from build123d import *
from build123d.topology import SkipClean

# Parameters (mm, degrees)
SKETCH_1_R          = 1
EXTRUDE_1_DEPTH     = 3
SKETCH_2_R          = 1
EXTRUDE_2_DEPTH     = 3
EXTRUDE_START       = -3
SKETCH_2_5_R        = 1
EXTRUDE_4_DEPTH     = 3.5
SKETCH_1_6_R        = 1.75
CUT_EXTRUDE_2_DEPTH = 4.5


with BuildPart() as part:
    # 草图1 → 凸台-拉伸1 (new body)
    with BuildSketch(Plane.XY):
        with BuildLine():
            Line((-16.25, -32.145825623), (16.25, -32.145825623))
            ThreePointArc((16.25, -32.145825623), (20.25, -28.145825623), (16.25, -24.145825623))
            Line((16.25, -24.145825623), (0, -24.145825623))
            Line((0, -24.145825623), (-16.25, -24.145825623))
            ThreePointArc((-16.25, -24.145825623), (-20.25, -28.145825623), (-16.25, -32.145825623))
        make_face()
        with Locations((-16.25, -28.145825623)):
            Circle(SKETCH_1_R, mode=Mode.SUBTRACT)
        with Locations((16.25, -28.145825623)):
            Circle(SKETCH_1_R, mode=Mode.SUBTRACT)
    extrude(amount=EXTRUDE_1_DEPTH)

    # 草图2 → 凸台-拉伸2 (add)
    with BuildSketch(Plane(origin=(0, 0, 0), x_dir=(-1, 0, 0), z_dir=(0, 0, -1))):
        with BuildLine():
            ThreePointArc((-16.356032043, -101.464832065), (-12.998767478, -105.201322829), (-8.636789042, -102.71019202))
            Line((-8.636789042, -102.71019202), (19.97488875, -29.603633498))
            ThreePointArc((19.97488875, -29.603633498), (14.792192125, -31.870714373), (12.52511125, -26.688017748))
            Line((12.52511125, -26.688017748), (-8.745712257, -81.037738685))
            Line((-8.745712257, -81.037738685), (-9.274078909, -83.991512561))
            Line((-9.274078909, -83.991512561), (-12.255645749, -27.933377702))
            ThreePointArc((-12.255645749, -27.933377702), (-16.037552079, -32.140179874), (-20.244354251, -28.358273544))
            Line((-20.244354251, -28.358273544), (-16.356032043, -101.464832065))
        make_face()
        with Locations((-12.361677792, -101.252384145)):
            Circle(SKETCH_2_R, mode=Mode.SUBTRACT)
    extrude(amount=-EXTRUDE_2_DEPTH)

    # 草图2<5> → 凸台-拉伸4 (add)
    # profile 1 of 2: a face of its own
    with SkipClean():  # the faces are left unmerged after this step: merging them gives an invalid solid
        with BuildSketch(Plane(origin=(0, 0, 0), x_dir=(-1, 0, 0), z_dir=(0, 0, -1)).offset(EXTRUDE_START)):
            with BuildLine():
                ThreePointArc((-16.25, -24.145825623), (-19.152567112, -25.393534912), (-20.244354251, -28.358273544))
                ThreePointArc((-20.244354251, -28.358273544), (-19.002290711, -31.048392735), (-16.25, -32.145825623))
                ThreePointArc((-16.25, -32.145825623), (-13.421572875, -30.974252748), (-12.25, -28.145825623))
                ThreePointArc((-12.25, -28.145825623), (-12.251411686, -28.039564161), (-12.255645749, -27.933377702))
                ThreePointArc((-12.255645749, -27.933377702), (-13.497709289, -25.243258511), (-16.25, -24.145825623))
            make_face()
            with Locations(Location((-16.25, -28.145825623, 0), (0, 0, 180))):
                Circle(SKETCH_2_5_R, mode=Mode.SUBTRACT)
        # profile 2 of 2: a face of its own
        with BuildSketch(Plane(origin=(0, 0, 0), x_dir=(-1, 0, 0), z_dir=(0, 0, -1)).offset(EXTRUDE_START)):
            with BuildLine():
                ThreePointArc((16.25, -32.145825623), (18.504857922, -31.449704518), (19.97488875, -29.603633498))
                ThreePointArc((19.97488875, -29.603633498), (20.180620498, -28.887595466), (20.25, -28.145825623))
                ThreePointArc((20.25, -28.145825623), (19.078427125, -25.317398498), (16.25, -24.145825623))
                ThreePointArc((16.25, -24.145825623), (13.995142078, -24.841946728), (12.52511125, -26.688017748))
                ThreePointArc((12.52511125, -26.688017748), (12.946121105, -30.400683545), (16.25, -32.145825623))
            make_face()
            with Locations(Location((16.25, -28.145825623, 0), (0, 0, 180))):
                Circle(SKETCH_2_5_R, mode=Mode.SUBTRACT)
        extrude(amount=-EXTRUDE_4_DEPTH)

    # 草图1<6> → 切除-拉伸2 (cut)
    with SkipClean():  # the faces are left unmerged after this step: merging them gives an invalid solid
        with BuildSketch(Plane.XY):
            with Locations((-16.25, -28.145825623)):
                Circle(SKETCH_1_6_R)
            with Locations((16.25, -28.145825623)):
                Circle(SKETCH_1_6_R)
        extrude(amount=CUT_EXTRUDE_2_DEPTH, mode=Mode.SUBTRACT)


solid = part.part
Input: part model. Units: mm. Frame: model coordinates. A direction names the side the tool comes from. Coordinates: 2 decimals unless noted, no trailing zeros. Write each loop counter-clockwise with the first axis right and the second up, starting at its lowest first coordinate (ties: lowest second). Pieces come first, ordered by that corner, then holes. Notation, with made-up numbers: M 89.5,-28.75 L 145.5,-28.75 A28 cw 145.5,-7.75 Z; hole C 1.25,24.25 d10. An arc over 180 degrees is marked long. Answer as a JSON object with one key per item and string values. Group by question number.
(1) Section B-B on x = -9. Output: boundary loops of the cut face in (y, z).
(2) Set-up query: faces 1 (the face through (16.02, -26.41, 2.22)), 2 (the face through (18.327, -64.4, 1.479)), 3 (the face through (10.634, -58.432, 1.479)). Return all of +Z, -Z, +X, -X, +Y, -Y with unobstructed straight access to the full face (end or side cutting, diameter ignored); none if empty.
(3) Contact query for flat-ended pins moving along their axis: P1, Ø3, axis at x = -16.25, y = -28.15, coming from the -Z side; P2, Ø2, axis at x = -2, y = -57.5, coming from the +Z side; P3, Ø2, axis at y = -85, z = 2.5, coming from the +X side. Output: stop coordinate, or through.
(4) Section C-C on y = -86.5. Output: boundary loops of the cut face in (x, z), plus the area to 3 significant figures.
(5) Ray query, line 1 along Y through (x, z) = (16.25, 5.3); line 2 along Z through (x, y) = (1, -80); line 3 along X through (y, z) = (-55.5, 2.5). Return the intervals inside material, ascending. Write a range as [from, to].
(6) Section A-A on y = -34. Output: boundary loops of the cut face in (x, z).
(7) Mould query, pull axis Y, two halves, no side actions, for faces 4 (the face through (13.07, -105.19, 1.48)), 5 (the face through (-15.79, -27.26, 5.49)), 6 (the face through (15, -29, 6.5)). Classes: pulls with the +Y half, pulls with the -Y half, needs draft (parallel to the pull), parting line crosses it, or undercut.
Result set:
{
 "1": {"outline": "M -57.65,0 L -35.7,0 L -35.7,3 L -57.65,3 Z; M -32.15,0 L -24.15,0 L -24.15,3 L -32.15,3 Z"},
 "2": {"face 1": "-Z", "face 2": "+Z, -Z, +X, -Y", "face 3": "+Z, -Z"},
 "3": {"P1": "stops at z = 4.5", "P2": "stops at z = 3", "P3": "stops at x = 17.28"},
 "4": {"outline": "M 2.29,0 L 17.15,0 L 17.15,3 L 2.29,3 Z", "area": "44.6 mm2"},
 "5": {"line 1": "y = [-32.15, -29.15], [-27.15, -24.15]", "line 2": "z = [0, 3]", "line 3": "x = [-9.84, -1.25], [10.79, 18.8]"},
 "6": {"outline": "M -18.25,0 L -9.66,0 L -9.66,3 L -18.25,3 Z; M 11.93,0 L 19.94,0 L 19.94,3 L 11.93,3 Z"},
 "7": {"face 4": "pulls with the -Y half", "face 5": "undercut", "face 6": "needs draft"}
}
